Read the model definition and answer for the solid it produces. Units are mm, in the model's axes. Coordinates: 2 decimals unless noted, no trailing zeros. Order: outer loops, then holes, each group sorted by start corner. A loop starts at its lowest first (then second) coordinate and runs counter-clockwise, first axis right, second up. Notation, with made-up numbers: (22, 39.25) -> (64, 39.25) arc R30 ccw to (64, 74.25) -> close; hole circle Ø9 at (-16, 34.5). An arc over 180 degrees is marked (long way). Answer in a Markdown table with one row per item.
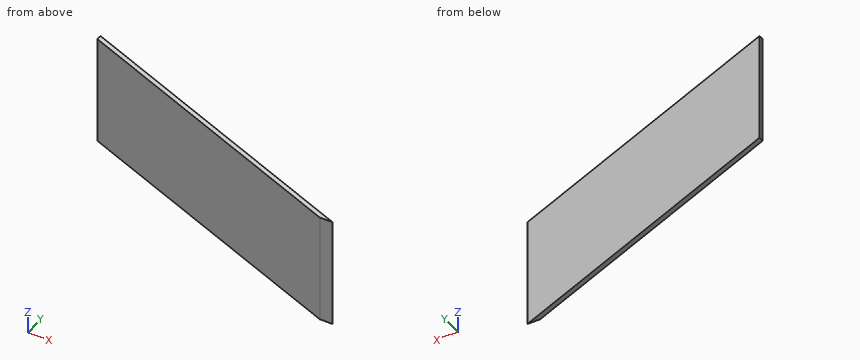
from build123d import *

# Parameters (mm, degrees)
F0_W     = 190.5
F0_H     = 76.2
F1_DEPTH = 66.675
F3_DEPTH = 76.2
F5_DEPTH = 76.2


with BuildPart() as f1:
    # F0 (on Top) → F1 (new body)
    with BuildSketch(Plane.XY):
        with Locations((95.25, 38.1)):
            Rectangle(F0_W, F0_H)
    extrude(amount=F1_DEPTH)

    # F2 (on face) → F3 (cut)
    with BuildSketch(Plane.XY.offset(66.675)):
        Polygon((0, 76.2), (190.5, 0), (190.5, 76.2), align=None)
    extrude(amount=-F3_DEPTH, mode=Mode.SUBTRACT)

    # F4 (on face) → F5 (cut)
    with BuildSketch(Plane.XY.offset(66.675)):
        Polygon((182.5625, 0), (0, 73.025), (0, 0), align=None)
    extrude(amount=-F5_DEPTH, mode=Mode.SUBTRACT)


solid = f1.part
Q1. The part is cut by section B-B (y = 31). Write down the section's boundary in (x, z) (1 decimal).
Outcome:
| item | result |
|---|---|
| outline | (105.1, 0) -> (113, 0) -> (113, 66.7) -> (105.1, 66.7) -> close |
Q2. Given pin 1 (1 mm diameter, centred on x = 140.5, z = 51.5, fed in from +Y); pin 2 (1 mm diameter, centred on x = 141, z = 59.5, fed in from +Y); pin 3 (8 mm diameter, centred on x = 162.5, z = 39.5, fed in from -Y) (3 decimals); pin 4 (6 mm diameter, centred on x = 47.5, y = 50.5, fed in from +Z), each flat-ended and moving along its own axis, determine where each tip first touches the part or whether it passes through.
Outcome:
| item | result |
|---|---|
| pin 1 | y = 20.2 |
| pin 2 | y = 20 |
| pin 3 | y = 6.425 |
| pin 4 | through |
Q3. The part is cut by section A-A (z = 57.5). Write down the section's boundary in (x, y) (1 decimal).
Outcome:
| item | result |
|---|---|
| outline | (0, 73) -> (182.6, 0) -> (190.5, 0) -> (0, 76.2) -> close |
Q4. Consider line 1 (Y direction, x = 43.5, z = 49.5) (3 decimals); line 2 (Y direction, x = 106.5, z = 13) (3 decimals). Determine where each line is inside the solid, lowest interval first.
Outcome:
| item | result |
|---|---|
| line 1 | 55.625 to 58.8 |
| line 2 | 30.425 to 33.6 |
